Geometry check sheet. Reference: the model listing, model coordinates, mm. A direction names the side the tool comes from. Round coordinates to 2 decimals unless told otherwise and drop trailing zeros. Order: outer loops, then holes, each group sorted by start corner. A loop starts at its lowest first (then second) coordinate and runs counter-clockwise, first axis right, second up. Notation, with made-up numbers: (44, 74) - (88, 74) arc R12 ccw to (88, 96) - close; hole circle Ø3 at (25.5, 57.25). An arc over 180 degrees is marked (long way). One line per question, with ' | ' between items. Start each with the question number.
Q1. Sectioned sample at A-A, the plane y = 21. Enter the section's corners in (x, z).
Q2. Tool access check on faces 5 (the face through (19.27, 20.96, -10.74)), 6 (the face through (29, 22, 1)), 7 (the face through (31.376, 23.507, 0.638)). Record the directions out of +Z, -Z, +X, -X, +Y, -Y that give a thin tool (end or side, any length) a straight path to the whole face; none if there is none.
Q3. Mould release check, pull along X, two halves, no side actions. Record for faces 1 (the face through (29, 25, -1)), 2 (the face through (7, -18, 0)), 3 (the face through (24.882, -0.231, 0.352)), 4 (the face through (28.89, 0.31, 0.02)): +X half, -X half, draft (parallel to the pull), parting line (faces both ways), or undercut.
Q4. Gauge pin test, flat ends, axial feed: P1, Ø2, axis at y = -14, z = -9, coming from the +X side; P2, Ø13, axis at x = 16.89, z = 0, coming from the -Y side; P3, Ø4, axis at y = -11, z = 8.5, coming from the -X side; P4, Ø11, axis at x = 14.5, z = 4.5, coming from the +Y side. Record the tip position at first contact, or that the pin passes through.
Q5. Material ranges on line 1 along Z through (x, y) = (16.89, 3.5); line 2 along Z through (x, y) = (16.89, 20.45); line 3 along X through (y, z) = (-6, -4.25), recorded low to high.
Q6. Sectioned sample at B-B, the plane y = -4. Enter the section's corners in (x, z), then the cut area to 3 significant figures.
```python
from build123d import *

# Parameters (mm, degrees)
CHAMFER_SIZE    = 1.5
SKETCH001_W     = 1.5
SKETCH001_H     = 3
SKETCH002_W     = 3
SKETCH002_H     = 44
GROOVE_ANGLE    = 20
FILLET_R        = 0.4
CHAMFER002_SIZE = 1


with BuildPart() as part:
    # Sketch → Revolution (revolve)
    with BuildSketch(Plane.XY):
        Polygon((-13, -25), (-13, 25), (-11, 25), (-11, 18), (-8, 18), (-8, -18), (-11, -18), (-11, -25), align=None)
    revolve(axis=Axis((0, 0, 0), (0, 1, 0)))

    # Chamfer
    chamfer_edges = [part.edges().sort_by_distance(p)[0] for p in [
        (8, -18, 0),
        (8, 18, 0),
    ]]
    chamfer(chamfer_edges, length=CHAMFER_SIZE)

    # Sketch001 → Revolution001 (revolve)
    with BuildSketch(Plane.XY):
        with Locations((-13.75, 23.5)):
            Rectangle(SKETCH001_W, SKETCH001_H)
    revolution001 = revolve(axis=Axis((0, 0, 0), (0, 1, 0)))

    # Mirrored: Revolution001 across XZ
    add(revolution001.mirror(Plane.XZ))

    # Sketch002 → Groove (revolve, symmetric, cut)
    with BuildSketch(Plane.XY) as groove_sk:
        with Locations((13.5, 0)):
            Rectangle(SKETCH002_W, SKETCH002_H)
    revolve(axis=Axis((0, 0, 0), (0, 1, 0)), revolution_arc=GROOVE_ANGLE / 2, mode=Mode.SUBTRACT)
    revolve(groove_sk.sketch, axis=Axis((0, 0, 0), (0, -1, 0)), revolution_arc=GROOVE_ANGLE / 2, mode=Mode.SUBTRACT)

    # Fillet
    fillet_edges = [part.edges().sort_by_distance(p)[0] for p in [
        (12.802501, 0, 2.257426),
        (12.802501, 0, -2.257426),
        (11.817693, 0, -2.083778),
        (11.817693, 0, 2.083778),
    ]]
    fillet(fillet_edges, radius=FILLET_R)

    # Chamfer002
    chamfer002_edges = [part.edges().sort_by_distance(p)[0] for p in [
        (14.5, 25, 0),
        (14.5, -25, 0),
        (11, 25, 0),
        (11, -25, 0),
        (-1.263758, 22, 14.444823),
        (-1.263758, -22, 14.444823),
    ]]
    chamfer(chamfer002_edges, length=CHAMFER002_SIZE)


with BuildPart() as part_1:
    # Body placement: moved
    add(part.part.moved(Location((16.89, 0, 0))))


solid = part_1.part
```
Determined:
1) outline: (28.77, -1.7) arc R12 ccw to (28.77, 1.7) arc R0.4 cw to (29.1, 2.15) - (29.29, 2.19) arc R0.4 ccw to (29.61, 2.66) arc R13 ccw (long way) to (29.61, -2.66) arc R0.4 ccw to (29.29, -2.19) - (29.1, -2.15) arc R0.4 cw to start; hole circle Ø22 at (16.89, 0)
2) face 5: +Y | face 6: none | face 7: +Y, -Y
3) face 1: draft | face 2: undercut | face 3: undercut | face 4: +X half
4) P1: stops at x = 27.14 | P2: passes through | P3: stops at x = 5.63 | P4: stops at y = 18
5) line 1: z = -13 to -8, 8 to 13 | line 2: z = -13 to -11, 11 to 13 | line 3: x = 4.6 to 10.11, 23.67 to 29.18
6) outline: (28.77, -1.7) arc R12 ccw to (28.77, 1.7) arc R0.4 cw to (29.1, 2.15) - (29.29, 2.19) arc R0.4 ccw to (29.61, 2.66) arc R13 ccw (long way) to (29.61, -2.66) arc R0.4 ccw to (29.29, -2.19) - (29.1, -2.15) arc R0.4 cw to start; hole circle Ø16 at (16.89, 0) | area: 325 mm2
